Autodesk Inventor part; units mm, degrees
ref_plane "YZ Plane" through (0, 0, 0) normal (1, 0, 0) x (0, 1, 0)
ref_plane "XZ Plane" through (0, 0, 0) normal (0, 1, 0) x (-1, 0, 0)
ref_plane "XY Plane" through (0, 0, 0) normal (0, 0, 1) x (1, 0, 0)
sketch "Sketch1" plane through (0, 0, 0) normal (0, 0, 1) x (1, 0, 0)
  line L0 (0, 0) -> (0, 6)
  line L1 (0, 6) -> (10, 6)
  line L2 (10, 6) -> (10, 0)
  line L3 (10, 0) -> (30, 0)
  line L4 (30, 0) -> (30, 6)
  line L5 (30, 6) -> (50, 6)
  line L6 (50, 6) -> (50, 0)
  line L7 (50, 0) -> (70, 0)
  line L8 (70, 0) -> (70, 6)
  line L9 (70, 6) -> (90, 6)
  line L10 (90, 6) -> (90, 1)
  line L11 (90, 1) -> (110, 1)
  line L12 (110, 1) -> (110, 6)
  line L13 (110, 6) -> (130, 6)
  line L14 (130, 6) -> (130, 1)
  line L15 (130, 1) -> (140, 1)
  line L16 (140, 1) -> (140, 6)
  line L17 (140, 6) -> (150, 6)
  line L18 (150, 6) -> (150, 316)
  line L19 (150, 316) -> (0, 316)
  line L20 (0, 316) -> (0, 6)
  circle A0 centre (110, 276) radius 30
  dimension "d0" = 6
  dimension "d1" = 10
  dimension "d2" = 20
  dimension "d3" = 20
  dimension "d4" = 20
  dimension "d5" = 20
  dimension "d6" = 20
  dimension "d7" = 20
  dimension "d8" = 10
  dimension "d9" = 10
  dimension "d10" = 310
  dimension "d13" = 60
  dimension "d14" = 40
  dimension "d16" = 40
extrude "Extrusion1" add sketch "Sketch1" against normal blind 6
properties part number "Exit"
CAD build for the part. Positions are in the model's coordinates, mm. A direction names the side the tool comes from. Give positions to 0.01 mm unless a question says otherwise; leave off trailing zeros. Order: outer loops, then holes, each group sorted by start corner. A loop starts at its lowest first (then second) coordinate and runs counter-clockwise, first axis right, second up. Notation, with made-up numbers: (49, 20) - (87, 20) arc R16 ccw to (87, 41) - close; hole circle Ø10 at (46.5, 56). An arc over 180 degrees is marked (long way). Answer in a Markdown table with one row per item.
1. Tool access for faces 1 (the flat face through (10, 3, -3)), 2 (the flat face through (40, 6, -3)), 3 (the flat face through (100, 1, -3)), 4 (the flat face through (0, 163, -3)), 5 (the flat face through (60, 0, -3)): list every direction of +Z, -Z, +X, -X, +Y, -Y with a clear straight run to the whole face (end or side of a thin tool).
Data:
| item | result |
|---|---|
| face 1 | +Z, -Z, -X, -Y |
| face 2 | +Z, -Z, -Y |
| face 3 | +Z, -Z, +X, -Y |
| face 4 | +Z, -Z, -X, +Y, -Y |
| face 5 | +Z, -Z, +X, -X, -Y |
2. Probe probe 1 along Y at (x, z) = (103, -5.6). List the from-to ranges inside material, lowest first. Write a range as [from, to].
Data:
| item | result |
|---|---|
| probe 1 | y = [1, 246.83], [305.17, 316] |
3. Pull direction X, two halves, no side cores. Call faces 6 (the cylindrical face through (103.497, 246.713, -2.958)), 7 (the flat face through (135, 1, -3)), 8 (the flat face through (150, 159, -3)): pulls with the +X half, pulls with the -X half, needs draft (parallel to the pull), parting line crosses it, or undercut.
Data:
| item | result |
|---|---|
| face 6 | undercut |
| face 7 | needs draft |
| face 8 | pulls with the +X half |
4. Saw through at C-C, the plane x = 76. Give the cut face in (y, z).
Data:
| item | result |
|---|---|
| outline | (6, -6) - (316, -6) - (316, 0) - (6, 0) - close |
5. Flat gauge pins, fed straight in: pin 1 (1.8 mm diameter, centred on x = 100.5, z = -3, fed in from -Y); pin 2 (2.5 mm diameter, centred on y = 4, z = -2, fed in from -X); pin 3 (1.8 mm diameter, centred on x = 116, z = -1.5, fed in from -Y). Where does each tip first touch, or does it go through?
Data:
| item | result |
|---|---|
| pin 1 | stops at y = 1 |
| pin 2 | stops at x = 10 |
| pin 3 | stops at y = 6 |
6. Saw through at B-B, the plane z = -3.15. Give the cut face in (x, y).
Data:
| item | result |
|---|---|
| outline | (0, 6) - (10, 6) - (10, 0) - (30, 0) - (30, 6) - (50, 6) - (50, 0) - (70, 0) - (70, 6) - (90, 6) - (90, 1) - (110, 1) - (110, 6) - (130, 6) - (130, 1) - (140, 1) - (140, 6) - (150, 6) - (150, 316) - (0, 316) - close; hole circle Ø60 at (110, 276) |
7. Saw through at A-A, the plane y = 276. Give the cut face in (x, z), plus the area to 3 significant figures.
Data:
| item | result |
|---|---|
| outline | (0, -6) - (80, -6) - (80, 0) - (0, 0) - close; (140, -6) - (150, -6) - (150, 0) - (140, 0) - close |
| area | 540 mm² |
